Read the model definition and answer for the solid it produces. Units are mm, in the model's axes. A direction names the side the tool comes from. Coordinates: 2 decimals unless noted, no trailing zeros. Write each loop counter-clockwise with the first axis right and the second up, starting at its lowest first coordinate (ties: lowest second). Pieces come first, ordered by that corner, then holes. Notation, with made-up numbers: (58, 78) -> (68, 78) arc R18 cw to (68, 105) -> close; hole circle Ø10 at (9.5, -11.75). An arc over 180 degrees is marked (long way). Answer as a JSON object with one key per item and string values. Group by question number.
(1) Straight lines are drawn through the part: L1, parallel to X at y = 10, z = -31; L2, parallel to Z at x = 90, y = 8.25; L3, parallel to Z at x = 17.25, y = 4.5. For each, find the intervals that lie inside material, in ascending order.
(2) Find section D-D (z = -184.5). Give the vertices of the cut face in (x, y), then the cut area to 3 significant figures.
(3) Flat-ended cylindrical pins translate along their axes: P1, Ø6, axis at x = 143.5, y = 10, coming from the +Z side; P2, Ø3, axis at y = 12.5, z = -73, coming from the +X side; P3, Ø7.5, axis at x = 63.5, z = -99.5, coming from the +Y side; P4, Ø10, axis at x = 129, y = 10.5, coming from the -Z side. Find the tip coordinate at first contact, or state that the pin passes through.
(4) Find section B-B (z = -97.5). Give the vertices of the cut face in (x, y), then the cut area to 3 significant figures.
(5) Find section A-A (x = 61.25). Give the vertices of the cut face in (y, z), then the cut area to 3 significant figures.
(6) Find section C-C (x = 17.25). Give the vertices of the cut face in (y, z).
(7) Which of the six approach directions +Z, -Z, +X, -X, +Y, -Y give full straight-line access (tool end or side, diameter ignored) to faces 1 (the face through (72, 5, -110)), 2 (the face through (75, 10, -98)), 3 (the face through (79, 8, -11))?
(8) For a pull along X with two mould halves and no side action, classify faces 4 (the face through (24.681, 6.984, -11.281)), 5 (the face through (77, 5, 0)), 6 (the face through (0, 10, -97)) as +X half, -X half, draft (parallel to the pull), parting line (faces both ways), or undercut.
from build123d import *

# Parameters (mm, degrees)
LINEAR_AUSTRAGEN1_DEPTH              = 20
LINEAR_AUSTRAGEN2_DEPTH              = 10
F_12_0_12_DURCHMESSER_BOHRUNG1_D     = 12
F_12_0_12_DURCHMESSER_BOHRUNG1_DEPTH = 25
F_10_0_10_DURCHMESSER_BOHRUNG1_D     = 10
M6_GEWINDEBOHRUNG1_REACH             = 154.5
M6_GEWINDEBOHRUNG1_BORE_R            = 2.5
M8_GEWINDEBOHRUNG1_D                 = 6.8
M8_GEWINDEBOHRUNG1_DEPTH             = 22.25
M8_GEWINDEBOHRUNG1_TIP               = 2.042926105
M6_GEWINDEBOHRUNG3_D                 = 5
M6_GEWINDEBOHRUNG3_DEPTH             = 17
M6_GEWINDEBOHRUNG3_TIP               = 1.502151548
M8_GEWINDEBOHRUNG2_D                 = 6.8
M8_GEWINDEBOHRUNG2_DEPTH             = 22.25
M8_GEWINDEBOHRUNG2_TIP               = 2.042926105


with BuildPart() as part:
    # Skizze1 → Linear austragen1 (new body)
    with BuildSketch(Plane(origin=(0, 0, 0), x_dir=(1, 0, 0), z_dir=(0, 1, 0))):
        with BuildLine():
            Line((0, 0), (0, 196))
            ThreePointArc((0, 196), (2.928932188, 203.071067812), (10, 206))
            Line((10, 206), (102.75, 206))
            Line((102.75, 206), (102.75, 181))
            Line((102.75, 181), (42.75, 181))
            ThreePointArc((42.75, 181), (35.678932188, 178.071067812), (32.75, 171))
            Line((32.75, 171), (32.75, 120))
            ThreePointArc((32.75, 120), (35.678932188, 112.928932188), (42.75, 110))
            Line((42.75, 110), (102.75, 110))
            Line((102.75, 110), (102.75, 45))
            ThreePointArc((102.75, 45), (105.678932188, 37.928932188), (112.75, 35))
            Line((112.75, 35), (152.5, 35))
            Line((152.5, 35), (152.5, 0))
            Line((152.5, 0), (102.75, 0))
            Line((102.75, 0), (0, 0))
        make_face()
    extrude(amount=LINEAR_AUSTRAGEN1_DEPTH)

    # Skizze20 → Linear austragen2 (cut)
    with BuildSketch(Plane(origin=(0, 20, 0), x_dir=(1, 0, 0), z_dir=(0, 1, 0))):
        with BuildLine():
            Line((47.75, 110), (47.75, 95))
            ThreePointArc((47.75, 95), (50.678932188, 87.928932188), (57.75, 85))
            Line((57.75, 85), (102.75, 85))
            Line((102.75, 85), (102.75, 110))
            Line((102.75, 110), (47.75, 110))
        make_face()
    extrude(amount=-LINEAR_AUSTRAGEN2_DEPTH, mode=Mode.SUBTRACT)

    # Ø12.0 (12) Durchmesser Bohrung1
    with Locations(Plane(origin=(0, 0, -206), x_dir=(-1, 0, 0), z_dir=(0, 0, -1))):
        with Locations((-75.25, 10)):
            Hole(F_12_0_12_DURCHMESSER_BOHRUNG1_D / 2, depth=F_12_0_12_DURCHMESSER_BOHRUNG1_DEPTH)

    # Ø10.0 (10) Durchmesser Bohrung1 (through all)
    with Locations(Plane(origin=(51, 20, 10), x_dir=(1, 0, 0), z_dir=(0, 1, 0))):
        with Locations((-33.75, 85)):
            Hole(F_10_0_10_DURCHMESSER_BOHRUNG1_D / 2)

    # M6 Gewindebohrung1 bore → M6 Gewindebohrung1 (cut, up to next)
    with BuildSketch(Plane.ZY, mode=Mode.PRIVATE) as m6_gewindebohrung1_sk1:
        with Locations((-75, 10)):
            Circle(M6_GEWINDEBOHRUNG1_BORE_R)
    m6_gewindebohrung1_tool1 = extrude(m6_gewindebohrung1_sk1.sketch, amount=-M6_GEWINDEBOHRUNG1_REACH, mode=Mode.PRIVATE) & part.part
    add(m6_gewindebohrung1_tool1.solids().sort_by_distance((0, 10, -75))[0], mode=Mode.SUBTRACT)

    # M8 Gewindebohrung1
    with Locations(Plane(origin=(51.25, 10, 0), x_dir=(1, 0, 0), z_dir=(0, 0, 1))):
        with Locations((-25, 0), (25, 0)):
            Hole(M8_GEWINDEBOHRUNG1_D / 2, depth=M8_GEWINDEBOHRUNG1_DEPTH)
            with Locations((0, 0, -(M8_GEWINDEBOHRUNG1_DEPTH + M8_GEWINDEBOHRUNG1_TIP / 2))):  # 118° drill point
                Cone(0, M8_GEWINDEBOHRUNG1_D / 2, M8_GEWINDEBOHRUNG1_TIP, mode=Mode.SUBTRACT)

    # M6 Gewindebohrung3
    with Locations(Plane(origin=(6.209471485, 2.149988387, -35), x_dir=(-1, 0, 0), z_dir=(0, 0, -1))):
        with Locations((-137.290528515, 7.850011613), (-124.790528515, 7.850011613)):
            Hole(M6_GEWINDEBOHRUNG3_D / 2, depth=M6_GEWINDEBOHRUNG3_DEPTH)
            with Locations((0, 0, -(M6_GEWINDEBOHRUNG3_DEPTH + M6_GEWINDEBOHRUNG3_TIP / 2))):  # 118° drill point
                Cone(0, M6_GEWINDEBOHRUNG3_D / 2, M6_GEWINDEBOHRUNG3_TIP, mode=Mode.SUBTRACT)

    # M8 Gewindebohrung2
    with Locations(Plane(origin=(0, 10, 0), x_dir=(-1, 0, 0), z_dir=(0, 1, 0))):
        with Locations((-61.25, -97.5), (-89.25, -97.5)):
            Hole(M8_GEWINDEBOHRUNG2_D / 2, depth=M8_GEWINDEBOHRUNG2_DEPTH)
            with Locations((0, 0, -(M8_GEWINDEBOHRUNG2_DEPTH + M8_GEWINDEBOHRUNG2_TIP / 2))):  # 118° drill point
                Cone(0, M8_GEWINDEBOHRUNG2_D / 2, M8_GEWINDEBOHRUNG2_TIP, mode=Mode.SUBTRACT)


solid = part.part
Results below:
{
 "1": {"L1": "x = 0 to 128.5, 133.5 to 141, 146 to 152.5", "L2": "z = -206 to -181, -110 to -100.82, -94.18 to 0", "L3": "z = -206 to -80, -70 to 0"},
 "2": {"outline": "(0, 0) -> (102.75, 0) -> (102.75, 20) -> (0, 20) -> close; hole circle Ø12 at (75.25, 10)", "area": "1,940 mm2"},
 "3": {"P1": "stops at z = 0", "P2": "stops at x = 102.75", "P3": "stops at y = 10", "P4": "stops at z = -35"},
 "4": {"outline": "(0, 0) -> (57.85, 0) -> (57.85, 10) -> (47.75, 10) -> (47.75, 20) -> (0, 20) -> close; (64.65, 0) -> (85.85, 0) -> (85.85, 10) -> (64.65, 10) -> close; (92.65, 0) -> (102.75, 0) -> (102.75, 10) -> (92.65, 10) -> close", "area": "1,370 mm2"},
 "5": {"outline": "(0, -206) -> (20, -206) -> (20, -181) -> (0, -181) -> close; (0, -110) -> (10, -110) -> (10, -100.9) -> (0, -100.9) -> close; (0, -94.1) -> (10, -94.1) -> (10, -85) -> (20, -85) -> (20, 0) -> (0, 0) -> close", "area": "2,380 mm2"},
 "6": {"outline": "(0, -206) -> (20, -206) -> (20, -80) -> (0, -80) -> close; (0, -70) -> (20, -70) -> (20, 0) -> (0, 0) -> close"},
 "7": {"face 1": "+X, +Y, -Y", "face 2": "+X, +Y", "face 3": "+Z"},
 "8": {"face 4": "undercut", "face 5": "draft", "face 6": "-X half"}
}
